from build123d import *

# Parameters (mm, degrees)
SKETCH1_R           = 3.175
BOSS_EXTRUDE1_DEPTH = 127
CUT_EXTRUDE1_START  = -31.75
SKETCH2_W           = 1.117822334
SKETCH2_H           = 4.49012806
CUT_EXTRUDE1_DEPTH  = 63.5
SKETCH3_R           = 9.5
BOSS_EXTRUDE2_DEPTH = 6.35


with BuildPart() as part:
    # Sketch1 → Boss-Extrude1 (new body)
    with BuildSketch(Plane(origin=(0, 0, 0), x_dir=(1, 0, 0), z_dir=(0, 1, 0))):
        Circle(SKETCH1_R)
    extrude(amount=BOSS_EXTRUDE1_DEPTH)

    # Sketch2 → Cut-Extrude1 (cut)
    with BuildSketch(Plane.XZ.offset(CUT_EXTRUDE1_START)):
        with Locations((2.803975197, 0)):
            Rectangle(SKETCH2_W, SKETCH2_H)
    extrude(amount=-CUT_EXTRUDE1_DEPTH, mode=Mode.SUBTRACT)

    # Sketch3 → Boss-Extrude2 (add)
    with BuildSketch(Plane.XZ):
        Circle(SKETCH3_R)
    extrude(amount=BOSS_EXTRUDE2_DEPTH)


solid = part.part
Can you work these out from the model? Positions are in its coordinate system, mm. Coordinates: 2 decimals unless noted, no trailing zeros. Loops run counter-clockwise (first coordinate to the right, second up) from the corner with the lowest first, then second, coordinate; pieces in that order, holes last. Notation, with made-up numbers: M -13.75,12.25 L 27.25,12.25 A17 cw 27.25,28.25 Z; hole C 69.25,-21 d5. An arc over 180 degrees is marked long. Answer as CSV lines item,"result". Start each with the question number.
1. Suppose I cut it at C-C, the plane y = 41. List the corners of the cut face in (x, z) for me (3 decimals).
2. If I drill on probe 1 along Y at (x, z) = (-8.25, 4.5); probe 2 along X at (y, z) = (98.5, -2.75); probe 3 along X at (y, z) = (80, -1), over which ranges is the centre line in solid material (lowest first)? Write a range as [from, to].
3. Suppose I cut it at B-B, the plane x = 0. List the corners of the cut face in (y, z) for me (3 decimals), plus the area to 3 significant figures.
4. Suppose I cut it at A-A, the plane z = 0. List the corners of the cut face in (x, y) for me (3 decimals), plus the area to 3 significant figures.
5. For pin 1 Ø6 at (x, y) = (-4, 10.5) entering from -Z; pin 2 Ø3.5 at (y, z) = (71, -0.5) entering from +X; pin 3 Ø6 at (x, z) = (2, -5) entering from +Y; pin 4 Ø6 at (x, y) = (-2.5, 56) entering from +Z (3 decimals), each with a flat end and sliding along its axis, tell me the tip position at first contact or that it passes through.
6. Suppose I cut it at D-D, the plane y = 2. List the corners of the cut face in (x, z) for me (3 decimals), plus the area to 3 significant figures.
7. Thinking about a two-plate mould opening in Y: for faces 1 (the face through (2.245, 63, 0)), 2 (the face through (0, 127, 0)), 3 (the face through (0, -6.35, 0)), 4 (the face through (4.38, -3.13, -8.43)), which applies, +Y half, -Y half, draft (parallel to the pull), parting line (faces both ways), or undercut?
Output:
1,outline,"M 2.245,-2.245 L 2.245,2.245 A3.175 ccw long Z"
2,probe 1,"y = [-6.35, 0]"
2,probe 2,"x = [-1.59, 1.59]"
2,probe 3,"x = [-3.01, 2.25]"
3,outline,"M -6.35,-9.5 L 0,-9.5 L 0,-3.175 L 127,-3.175 L 127,3.175 L 0,3.175 L 0,9.5 L -6.35,9.5 Z"
3,area,"927 mm^2"
4,outline,"M -9.5,-6.35 L 9.5,-6.35 L 9.5,0 L 3.175,0 L 3.175,31.75 L 2.245,31.75 L 2.245,95.25 L 3.175,95.25 L 3.175,127 L -3.175,127 L -3.175,0 L -9.5,0 Z"
4,area,"868 mm^2"
5,pin 1,"stops at z = -3.01"
5,pin 2,"stops at x = 2.25"
5,pin 3,"stops at y = 127"
5,pin 4,"stops at z = 3.175"
6,outline,"C 0,0 d6.35"
6,area,"31.7 mm^2"
7,face 1,"undercut"
7,face 2,"+Y half"
7,face 3,"-Y half"
7,face 4,"draft"
